from build123d import *

# Parameters (mm, degrees)
F0_W         = 60
F0_H         = 18.8
F2_DEPTH     = 2
F3_DEPTH     = 3
F5_T1_DEPTH  = 30.5361420581
F6_SIZE2     = 5.494945
F6_SIZE      = 1.99999
F7_T1_DEPTH  = 59.3887824638
F7_T3_DEPTH  = 59.3938374638
F7_T5_DEPTH  = 22.4213203436
F7_T7_DEPTH  = 10.7363912706
F7_T9_DEPTH  = 3.6213303413
F7_T11_DEPTH = 12.745712209
F7_T13_DEPTH = 10.7363785984
F7_T15_DEPTH = 12.740667054
F7_T18_ANGLE = 180
F8_R         = 0.9656854249


# Not quite as in the source:
# - a fillet or chamfer that OpenCascade refuses, or shapes differently, is made with other operations: its cross-section is extruded or revolved along the edge and cut away or added
# - a fillet or chamfer is up to 0.001 mm smaller than in the source, because OpenCascade refuses the exact size


with BuildPart() as f2:
    # F0 (on Top) → F2 (new body)
    with BuildSketch(Plane.XY):
        Rectangle(F0_W, F0_H)
    extrude(amount=F2_DEPTH)


with BuildPart() as f3:
    # F1 (on Top) → F3 (new body)
    with BuildSketch(Plane.XY):
        with BuildLine():
            ThreePointArc((-19.0649479628, -7.3999999978), (-13.832357782, -5.2325901785), (-11.6649479628, 2.2e-09))
            ThreePointArc((-11.6649479628, 2.2e-09), (-13.832357782, 5.232590183), (-19.0649479628, 7.4000000022))
            Line((-19.0649479628, 7.4000000022), (-19.0649479628, -7.3999999978))
        make_face()
        with BuildLine():
            Line((-19.0649479628, -7.3999999978), (-19.0649479628, 7.4000000022))
            ThreePointArc((-19.0649479628, 7.4000000022), (-26.4649479628, 2.2e-09), (-19.0649479628, -7.3999999978))
        make_face()
        with BuildLine():
            ThreePointArc((-19.0649479628, -7.3999999978), (-26.4649479628, 2.2e-09), (-19.0649479628, 7.4000000022))
            Line((-19.0649479628, 7.4000000022), (-58.9926913381, 7.4000000022))
            Line((-58.9926913381, 7.4000000022), (-58.9926913381, -7.3999999978))
            Line((-58.9926913381, -7.3999999978), (-19.0649479628, -7.3999999978))
        make_face()
    extrude(amount=F3_DEPTH)


with BuildPart() as f2_1:
    add(f2.part)

    # F4: cut F3
    add(f3.part, mode=Mode.SUBTRACT)

    # F5: chamfer of 5.5 x 2.0018362885 on 1 edges, made by hand

    # F5_s2 → F5_t1 (cut)
    with BuildSketch(Plane.XY.offset(-14.268071029)):
        Polygon((-24.5, -9.4), (-30, -7.3981637115), (-30, -9.4), align=None)
    extrude(amount=F5_T1_DEPTH, mode=Mode.SUBTRACT)

    # F6 (size 2 and 5.4949548389 in the source; OpenCascade refuses exactly that, so slightly less here)
    f6_edges = [f2_1.edges().sort_by_distance(p)[0] for p in [
        (-30, 9.4, 1),
    ]]
    f6_side = f2_1.faces().sort_by_distance((-30, 8.4, 1))[0]
    chamfer(f6_edges, length=F6_SIZE, length2=F6_SIZE2, reference=f6_side)

    # F7: fillet of radius 0.7242640687 on 9 edges, made by hand

    # F7_s2 → F7_t1 (cut)
    with BuildSketch(Plane.YZ.offset(-27.578122292)):
        with BuildLine():
            ThreePointArc((-8.6757359313, 2), (-9.1878679656, 1.7878679656), (-9.4, 1.2757359313))
            Line((-9.4, 1.2757359313), (-9.4, 2))
            Line((-9.4, 2), (-8.6757359313, 2))
        make_face()
    extrude(amount=F7_T1_DEPTH, mode=Mode.SUBTRACT)

    # F7_s4 → F7_t3 (cut)
    with BuildSketch(Plane.YZ.offset(-27.583177292)):
        with BuildLine():
            ThreePointArc((9.4, 1.2757359313), (9.1878679656, 1.7878679656), (8.6757359313, 2))
            Line((8.6757359313, 2), (9.4, 2))
            Line((9.4, 2), (9.4, 1.2757359313))
        make_face()
    extrude(amount=F7_T3_DEPTH, mode=Mode.SUBTRACT)

    # F7_s6 → F7_t5 (cut)
    with BuildSketch(Plane.XZ.offset(-11.2106601718)):
        with BuildLine():
            ThreePointArc((30, 1.2757359313), (29.7878679656, 1.7878679656), (29.2757359313, 2))
            Line((29.2757359313, 2), (30, 2))
            Line((30, 2), (30, 1.2757359313))
        make_face()
    extrude(amount=F7_T5_DEPTH, mode=Mode.SUBTRACT)

    # F7_s8 → F7_t7 (cut)
    with BuildSketch(Plane(origin=(-25.8093615097, 9.3938393551, 0), x_dir=(0, 0, 1), z_dir=(0.9396926208, -0.3420201433, 0))):
        with BuildLine():
            ThreePointArc((2, 16.4883400783), (1.7878679656, 17.0004721126), (1.2757359313, 17.212604147))
            Line((1.2757359313, 17.212604147), (2, 17.212604147))
            Line((2, 17.212604147), (2, 16.4883400783))
        make_face()
    extrude(amount=F7_T7_DEPTH, mode=Mode.SUBTRACT)

    # F7_s10 → F7_t9 (cut)
    with BuildSketch(Plane.XZ.offset(-9.2106701718)):
        with BuildLine():
            ThreePointArc((-29.2757359313, 2), (-29.7878679656, 1.7878679656), (-30, 1.2757359313))
            Line((-30, 1.2757359313), (-30, 2))
            Line((-30, 2), (-29.2757359313, 2))
        make_face()
    extrude(amount=F7_T9_DEPTH, mode=Mode.SUBTRACT)

    # F7_s12 → F7_t11 (cut)
    with BuildSketch(Plane.YZ.offset(-31.8106601718)):
        with BuildLine():
            ThreePointArc((8.1242640709, 2), (7.6121320366, 1.7878679656), (7.4000000022, 1.2757359313))
            Line((7.4000000022, 1.2757359313), (7.4000000022, 2))
            Line((7.4000000022, 2), (8.1242640709, 2))
        make_face()
    extrude(amount=F7_T11_DEPTH, mode=Mode.SUBTRACT)

    # F7_s14 → F7_t13 (cut)
    with BuildSketch(Plane(origin=(-25.8138396564, -9.3954391126, 0), x_dir=(0, 0, 1), z_dir=(0.9396929736, 0.342019174, 0))):
        with BuildLine():
            ThreePointArc((1.2757359313, -17.2143126223), (1.7878679656, -17.0021805879), (2, -16.4900485536))
            Line((2, -16.4900485536), (2, -17.2143126223))
            Line((2, -17.2143126223), (1.2757359313, -17.2143126223))
        make_face()
    extrude(amount=F7_T13_DEPTH, mode=Mode.SUBTRACT)

    # F7_s16 → F7_t15 (cut)
    with BuildSketch(Plane.YZ.offset(-31.8056150167)):
        with BuildLine():
            ThreePointArc((-8.1242640665, 2), (-7.6121320321, 1.7878679656), (-7.3999999978, 1.2757359313))
            Line((-7.3999999978, 1.2757359313), (-7.3999999978, 2))
            Line((-7.3999999978, 2), (-8.1242640665, 2))
        make_face()
    extrude(amount=F7_T15_DEPTH, mode=Mode.SUBTRACT)

    # F7_s17 → F7_t18 (revolve, cut)
    with BuildSketch(Plane.YZ.offset(-19.0649479628)):
        with BuildLine():
            ThreePointArc((8.1242640709, 2), (7.6121320366, 1.7878679656), (7.4000000022, 1.2757359313))
            Line((7.4000000022, 1.2757359313), (7.4000000022, 2))
            Line((7.4000000022, 2), (8.1242640709, 2))
        make_face()
    revolve(axis=Axis((-19.0649479628, 2.2e-09, 2), (0, 0, -1)), revolution_arc=F7_T18_ANGLE, mode=Mode.SUBTRACT)

    # F8
    f8_edges = [f2_1.edges().sort_by_distance(p)[0] for p in [
        (2.75, -9.4, 0),
        (30, 0, 0),
        (2.747473, 9.4, 0),
    ]]
    fillet(f8_edges, radius=F8_R)


solid = f2_1.part
For this review, take the finished solid that the model builds, in its own axes (mm). A direction names the side the tool comes from. Round coordinates to 2 decimals unless told otherwise and drop trailing zeros. Order: outer loops, then holes, each group sorted by start corner. A loop starts at its lowest first (then second) coordinate and runs counter-clockwise, first axis right, second up. Notation, with made-up numbers: M 34,9 L 47,9 A21 cw 47,18 Z; hole C 86.5,33 d6. An arc over 180 degrees is marked long. Write each question's results on one line, items separated by ' | '. Start each with the question number.
1. Add section A-A (x = 21.5). State the section outline as (y, z) points, then the cut area to 3 significant figures.
2. Tool access review of faces 1 (the face through (-24, 7.4, 1)), 2 (the face through (-27.209, -8.414, 0.629)): name each direction out of +Z, -Z, +X, -X, +Y, -Y from which nothing blocks a thin tool from reaching the whole face with its end or side.
3. To check wall thickness, follow L1, parallel to X at y = 5, z = 1; L2, parallel to X at y = 4.75, z = 0.45; L3, parallel to Y at x = 11.5, z = 1.5. State the ranges of each line that lie inside material, in increasing order. Write a range as [from, to].
Output values:
1) outline: M -9.4,0.97 A0.97 ccw -8.43,0 L 8.43,0 A0.97 ccw 9.4,0.97 L 9.4,1.28 A0.72 ccw 8.68,2 L -8.68,2 A0.72 ccw -9.4,1.28 Z | area: 37.0 mm^2
2) face 1: +Z, -Z, -X | face 2: +Z, -Z, -X, -Y
3) L1: [-13.61, 30] | L2: [-13.39, 29.85] | L3: [-9.36, 9.36]
